The drawing under review shows one solid part. Ordinate dimensions are in mm from its lowest x, y, z. A direction names the side the tool comes from. Round coordinates to 2 decimals unless told otherwise and drop trailing zeros. Order: outer loops, then holes, each group sorted by start corner. A loop starts at its lowest first (then second) coordinate and runs counter-clockwise, first axis right, second up.
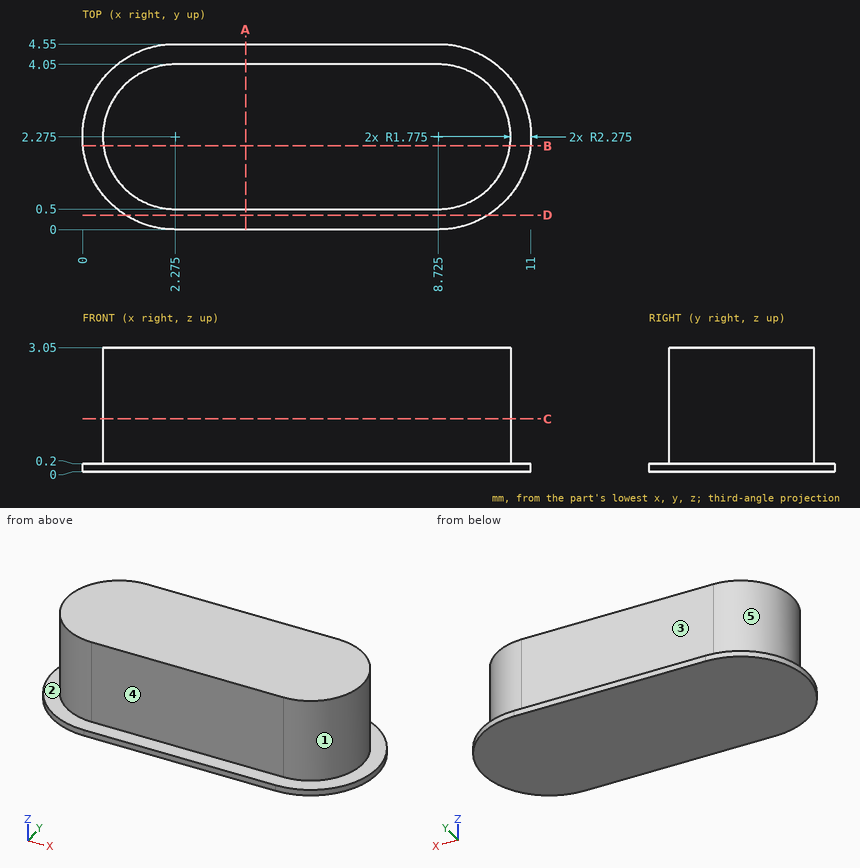
(1) To check wall thickness, follow L1, parallel to Z at x = 4.25, y = 0.4; L2, parallel to Y at x = 5.5, z = 0.65; L3, parallel to Y at x = 2, z = 0.15. State the ranges of each line that lie inside material, in increasing order.
(2) Clearance check with flat-ended pins moving along their axes: P1, Ø0.9, axis at x = 5, z = 1.5, coming from the -Y side; P2, Ø1, axis at x = 2.5, y = 1, coming from the -Z side; P3, Ø1.4, axis at x = 4, z = 2, coming from the +Y side; P4, Ø1.5, axis at y = 1, z = 2.5, coming from the -X side. State where each tip first meets the part, or that it passes through.
(3) We need section D-D (y = 0.35). Give the boundary of the cut face in (x, z).
(4) We need section C-C (z = 1.3). Give the boundary of the cut face in (x, y) (3 decimals).
(5) We need section B-B (y = 2.05). Give the boundary of the cut face in (x, z), and give its area (3 significant figures).
(6) We need section A-A (x = 4). Give the boundary of the cut face in (y, z), and give its area (3 significant figures).
(7) Tool access review of the marked faces 1, 2, 3, 4 and 5: name each direction out of +Z, -Z, +X, -X, +Y, -Y from which nothing blocks a thin tool from reaching the whole face with its end or side.
Verdict:
1. L1: z = 0 to 0.2
1. L2: y = 0.5 to 4.05
1. L3: y = 0.02 to 4.53
2. P1: stops at y = 0.5
2. P2: stops at z = 0
2. P3: stops at y = 4.05
2. P4: stops at x = 0.58
3. outline: (1.06, 0) - (9.94, 0) - (9.94, 0.2) - (1.06, 0.2) - close
4. outline: (2.275, 0.5) - (8.725, 0.5) arc R1.775 ccw to (8.725, 4.05) - (2.275, 4.05) arc R1.775 ccw to start
5. outline: (0.01, 0) - (10.99, 0) - (10.99, 0.2) - (10.49, 0.2) - (10.49, 3.05) - (0.51, 3.05) - (0.51, 0.2) - (0.01, 0.2) - close
5. area: 30.6 mm2
6. outline: (0, 0) - (4.55, 0) - (4.55, 0.2) - (4.05, 0.2) - (4.05, 3.05) - (0.5, 3.05) - (0.5, 0.2) - (0, 0.2) - close
6. area: 11.0 mm2
7. face 1: +Z, +X
7. face 2: +Z
7. face 3: +Z, +X, -X, +Y
7. face 4: +Z, +X, -X, -Y
7. face 5: +Z, -X
